The model under review builds one solid part; all positions refer to its coordinate system, in mm. Coordinates: 2 decimals unless noted, no trailing zeros. Write each loop counter-clockwise with the first axis right and the second up, starting at its lowest first coordinate (ties: lowest second). Pieces come first, ordered by that corner, then holes. Notation, with made-up numbers: M -39.75,20.25 L -35.75,20.25 A17 cw -35.75,49.25 Z; hole C 89,37.5 d8. An arc over 180 degrees is marked long. Answer as a JSON object with one key per item and string values.
```python
from build123d import *

# Parameters (mm, degrees)
PAD_DEPTH    = 2000
SKETCH001_R  = 140
POCKET_DEPTH = 50.001
CHAMFER_SIZE = 10


with BuildPart() as part:
    # Sketch → Pad (new body)
    with BuildSketch(Plane.XZ):
        with BuildLine():
            ThreePointArc((0, 25), (-25, 0), (0, -25))
            Line((0, -25), (550, -25))
            ThreePointArc((550, -25), (575, 0), (550, 25))
            Line((0, 25), (550, 25))
        make_face()
    extrude(amount=PAD_DEPTH)

    # Sketch001 (on Face4 of Pad) → Pocket (cut, through all)
    with BuildSketch(Plane(origin=(0, 0, 25), x_dir=(-1, 0, 0), z_dir=(0, 0, 1))):
        with Locations((-275, 1750)):
            Circle(SKETCH001_R)
        with Locations((-275, 1000)):
            Circle(SKETCH001_R)
        with Locations((-275, 250)):
            Circle(SKETCH001_R)
    extrude(amount=-POCKET_DEPTH, mode=Mode.SUBTRACT)

    # Chamfer
    chamfer_edges = [part.edges().sort_by_distance(p)[0] for p in [
        (415, -1750, 25),
        (415, -1000, 25),
        (415, -250, 25),
    ]]
    chamfer(chamfer_edges, length=CHAMFER_SIZE)


solid = part.part
```
(1) Wall thickness on line 1 along Y through (x, z) = (275, -7); line 2 along Y through (x, z) = (244.5, -22); line 3 along X through (y, z) = (-250, 4): over which ranges is each line inside the solid? List them lowest first. Write a range as from..to.
Results list:
{"line 1": "-2000..-1890, -1610..-1140, -860..-390, -110..0", "line 2": "-2000..-1886.64, -1613.36..-1136.64, -863.36..-386.64, -113.36..0", "line 3": "-24.68..135, 415..574.68"}
(2) For pin 1 Ø6 at (y, z) = (-1667.5, -13) entering from +X; pin 2 Ø8 at (x, z) = (397, 14) entering from +Y; pin 3 Ø6 at (y, z) = (-274, 9.5) entering from +X; pin 4 Ø1 at (y, z) = (-837.5, 15) entering from +X, all flat-tipped, find the tip position at first contact; note any pin that passes through.
Results list:
{"pin 1": "x = 572.91", "pin 2": "y = 0", "pin 3": "x = 574.14", "pin 4": "x = 570.37"}
(3) Add section C-C on x = 177.5. Count the separate pieces of the cut face and the enclosed holes in it, and give its area (4 significant figures).
Results list:
{"separate pieces": "4", "enclosed holes": "0", "area": "69,450 mm²"}
(4) Draft analysis for pull direction X (two halves, no side actions). For faces 1 (the face through (-24.994, -986, 0.55)), 2 (the face through (293.23, -1138.81, -4.72)), 3 (the face through (88, -986, -25)), 4 (the face through (199.74, -368.05, -4.72)), state which applies: released by +X, released by -X, zero draft, split by the parting line, or undercut.
Results list:
{"face 1": "released by -X", "face 2": "undercut", "face 3": "zero draft", "face 4": "undercut"}
(5) Add section D-D on y = -428. Give the boundary of the cut face in (x, z), and give its area (3 significant figures).
Results list:
{"outline": "M 0,-25 L 550,-25 A25 ccw 550,25 L 0,25 A25 ccw Z", "area": "29,500 mm²"}
(6) Add section B-B on z = 1.5. Give the boundary of the cut face in (x, y).
Results list:
{"outline": "M -24.95,-2000 L 574.95,-2000 L 574.95,0 L -24.95,0 Z; hole C 275,-1750 d280; hole C 275,-1000 d280; hole C 275,-250 d280"}
(7) Add section A-A on y = -1750. Give the boundary of the cut face in (x, z).
Results list:
{"outline": "M 0,-25 L 135,-25 L 135,15 L 125,25 L 0,25 A25 ccw Z; M 415,-25 L 550,-25 A25 ccw 550,25 L 425,25 L 415,15 Z"}
